```python
from build123d import *

# Parameters (mm, degrees)
BOSS_EXTRUDE1_DEPTH = 1.5
BOSS_EXTRUDE2_DEPTH = 1
SKETCH4_R           = 4.75
CUT_EXTRUDE1_DEPTH  = 23.898325822
SKETCH5_W           = 17.56
SKETCH5_H           = 2.5
BOSS_EXTRUDE3_DEPTH = 0.15
SKETCH6_W           = 17.56
SKETCH6_H           = 2.5
BOSS_EXTRUDE4_DEPTH = 7.5
SKETCH9_W           = 8
SKETCH9_H           = 2
CUT_EXTRUDE2_DEPTH  = 1
FILLET1_R           = 1
CUT_EXTRUDE3_REACH  = 30.47
SKETCH10_W          = 6.92
SKETCH10_H          = 1
SKETCH11_W          = 2.5
SKETCH11_H          = 3.588872583
CUT_EXTRUDE4_DEPTH  = 0.25


with BuildPart() as part:
    # Sketch1 → Boss-Extrude1 (new body)
    with BuildSketch(Plane.XY):
        with BuildLine():
            ThreePointArc((14.980604809, 6.55), (8.78, 2), (2.579395191, 6.55))
            Line((2.579395191, 6.55), (0, 6.55))
            Line((0, 6.55), (0, 0))
            Line((0, 0), (17.56, 0))
            Line((17.56, 0), (17.56, 6.55))
            Line((17.56, 6.55), (14.980604809, 6.55))
        make_face()
        with BuildLine():
            ThreePointArc((2.579395191, 6.55), (2.679421093, 10.743420825), (5.32, 14.002581212))
            Line((5.32, 14.002581212), (5.32, 14.619498126))
            ThreePointArc((5.32, 14.619498126), (1.449679407, 11.382680416), (0, 6.55))
            Line((0, 6.55), (2.579395191, 6.55))
        make_face()
        with BuildLine():
            ThreePointArc((12.24, 14.002581212), (14.880578907, 10.743420825), (14.980604809, 6.55))
            Line((14.980604809, 6.55), (17.56, 6.55))
            ThreePointArc((17.56, 6.55), (16.110320593, 11.382680416), (12.24, 14.619498126))
            Line((12.24, 14.619498126), (12.24, 14.002581212))
        make_face()
    extrude(amount=BOSS_EXTRUDE1_DEPTH)

    # Sketch3 → Boss-Extrude2 (add)
    with BuildSketch(Plane.XY.offset(1.5)):
        with BuildLine():
            Line((12.24, 14.619498126), (12.24, 14.002581212))
            ThreePointArc((12.24, 14.002581212), (8.78, 2), (5.32, 14.002581212))
            Line((5.32, 14.002581212), (5.32, 14.619498126))
            ThreePointArc((5.32, 14.619498126), (1.449679407, 11.382680416), (0, 6.55))
            Line((0, 6.55), (0, 0))
            Line((0, 0), (17.56, 0))
            Line((17.56, 0), (17.56, 6.55))
            ThreePointArc((17.56, 6.55), (16.110320593, 11.382680416), (12.24, 14.619498126))
        make_face()
        with BuildLine():
            Line((5.32, 14.619498126), (12.24, 14.619498126))
            Line((12.24, 14.619498126), (12.24, 14.002581212))
            ThreePointArc((12.24, 14.002581212), (8.78, 2), (5.32, 14.002581212))
            Line((5.32, 14.002581212), (5.32, 14.619498126))
        make_face()
    extrude(amount=BOSS_EXTRUDE2_DEPTH)

    # Sketch4 → Cut-Extrude1 (cut, through all)
    with BuildSketch(Plane(origin=(0, 0, 1.5), x_dir=(-1, 0, 0), z_dir=(0, 0, -1))):
        with Locations((-8.78, 8.5)):
            Circle(SKETCH4_R)
    extrude(amount=-CUT_EXTRUDE1_DEPTH, mode=Mode.SUBTRACT)

    # Sketch5 → Boss-Extrude3 (add)
    with BuildSketch(Plane.XZ):
        with Locations((8.78, 1.25)):
            Rectangle(SKETCH5_W, SKETCH5_H)
    extrude(amount=BOSS_EXTRUDE3_DEPTH)

    # Sketch6 → Boss-Extrude4 (add)
    with BuildSketch(Plane.XZ.offset(0.15)):
        with Locations((8.78, 1.25)):
            Rectangle(SKETCH6_W, SKETCH6_H)
    extrude(amount=BOSS_EXTRUDE4_DEPTH)

    # Sketch9 → Cut-Extrude2 (cut)
    with BuildSketch(Plane.XY.offset(2.5)):
        with Locations((8.78, -5.353166831)):
            Rectangle(SKETCH9_W, SKETCH9_H)
    extrude(amount=-CUT_EXTRUDE2_DEPTH, mode=Mode.SUBTRACT)

    # Fillet1
    fillet1_edges = [part.edges().sort_by_distance(p)[0] for p in [
        (4.78, -5.353166831, 2.5),
        (12.78, -5.353166831, 2.5),
        (8.78, -4.353166831, 2.5),
    ]]
    fillet(fillet1_edges, radius=FILLET1_R - 0.0001)  # a hair under: the kernel refuses the full size

    # Sketch10 → Cut-Extrude3 (cut, up to next)
    with BuildSketch(Plane(origin=(0, 14.619498126, 0), x_dir=(1, 0, 0), z_dir=(0, 1, 0)), mode=Mode.PRIVATE) as cut_extrude3_sk1:
        with Locations((8.78, -2)):
            Rectangle(SKETCH10_W, SKETCH10_H)
    cut_extrude3_tool1 = extrude(cut_extrude3_sk1.sketch, amount=-CUT_EXTRUDE3_REACH, mode=Mode.PRIVATE) & part.part
    add(cut_extrude3_tool1.solids().sort_by_distance((8.78, 14.619498, 2))[0], mode=Mode.SUBTRACT)

    # Sketch11 → Cut-Extrude4 (cut)
    with BuildSketch(Plane(origin=(5.32, 0, 0), x_dir=(0, 0, -1), z_dir=(1, 0, 0))):
        with Locations((-1.25, 12.825061835)):
            Rectangle(SKETCH11_W, SKETCH11_H)
    cut_extrude4 = extrude(amount=-CUT_EXTRUDE4_DEPTH, mode=Mode.SUBTRACT)

    # Mirror1: Cut-Extrude4 across plane
    add(cut_extrude4.mirror(Plane.ZY.offset(-8.78)), mode=Mode.SUBTRACT)


solid = part.part
```
For this review, take the finished solid that the model builds, in its own axes (mm). A direction names the side the tool comes from. Round coordinates to 2 decimals unless told otherwise and drop trailing zeros. Write each loop counter-clockwise with the first axis right and the second up, starting at its lowest first coordinate (ties: lowest second). Pieces come first, ordered by that corner, then holes. Notation, with made-up numbers: (5.25, 17) - (25.25, 17) arc R20 cw to (25.25, 31) - close; hole circle Ø1 at (89.5, -21.75). An arc over 180 degrees is marked (long way). Answer as CSV lines item,"result". Start each with the question number.
(1) Add section D-D, the plane y = 13. State the section outline as (x, z) points, plus the area to 3 significant figures.
(2) For line 1 (X direction, y = 8.5, z = 2.1); line 2 (Y direction, x = 8.78, z = 2.3); line 3 (Y direction, x = 8.78, z = 1.9), list the stretches that pass through material, from the lowest coordinate up.
(3) Mouldability with a two-part tool opening along Y and no side actions: class faces 4 (the flat face through (9, 1, 2.5)), 5 (the flat face through (9, -7.65, 1)), 6 (the cylindrical face through (13.081, -5.166, 2.215)) as +Y half, -Y half, draft (parallel to the pull), parting line (faces both ways), or undercut.
(4) Machinability: for faces 1 (the flat face through (12.49, 13, 2)), 2 (the flat face through (9, -5, 1.5)), 3 (the flat face through (8.7, 3.6, 1.5)), which of the approach directions +Z, -Z, +X, -X, +Y, -Y give a long, thin tool a straight path to every point of the face, cutting with its end or side? Answer none if there is none.
(5) Add section A-A, the plane y = 8.5. State the section outline as (x, z) points, plus the area to 3 significant figures.
(6) For pin 1 (1.1 mm diameter, centred on x = 11, z = 2, fed in from +Y); pin 2 (1.2 mm diameter, centred on y = 13, z = 1, fed in from -X); pin 3 (0.6 mm diameter, centred on x = 10.5, y = -5.5, fed in from +Z), all flat-tipped, find the tip position at first contact; note any pin that passes through.
(7) Add section B-B, the plane z = 0.5. State the section outline as (x, y) points.
From the geometry:
1,outline,"(2.82, 0) - (4.09, 0) - (4.09, 1.5) - (5.07, 1.5) - (5.07, 2.5) - (2.82, 2.5) - close; (12.49, 1.5) - (13.47, 1.5) - (13.47, 0) - (14.74, 0) - (14.74, 2.5) - (12.49, 2.5) - close"
1,area,"8.29 mm²"
2,line 1,"x = 0.22 to 4.03, 13.53 to 17.34"
2,line 2,"y = -7.65 to -6.35, -3.95 to 3.75"
2,line 3,"y = -7.65 to -6.35, -4.27 to 3.75"
3,face 4,"draft"
3,face 5,"-Y half"
3,face 6,"undercut"
4,face 1,"+Z, -Z, +Y"
4,face 2,"+Z"
4,face 3,"-Z"
5,outline,"(0.22, 0) - (2.28, 0) - (2.28, 1.5) - (4.03, 1.5) - (4.03, 2.5) - (0.22, 2.5) - close; (13.53, 1.5) - (15.28, 1.5) - (15.28, 0) - (17.34, 0) - (17.34, 2.5) - (13.53, 2.5) - close"
5,area,"13.8 mm²"
6,pin 1,"stops at y = 4.64"
6,pin 2,"stops at x = 2.23"
6,pin 3,"stops at z = 1.5"
7,outline,"(0, -7.65) - (17.56, -7.65) - (17.56, 6.55) arc R8.78 ccw to (12.49, 14.51) - (12.49, 13.84) arc R6.5 cw (long way) to (5.07, 13.84) - (5.07, 14.51) arc R8.78 ccw to (0, 6.55) - close"
